Could you check a few things on this model? Use its own coordinates, in mm. Give positions to 0.01 mm unless a question says otherwise; leave off trailing zeros. Write each loop counter-clockwise with the first axis right and the second up, starting at its lowest first coordinate (ties: lowest second). Pieces come first, ordered by that corner, then holes. Notation, with made-up numbers: (70.5, 68) -> (114.5, 68) arc R19 cw to (114.5, 79) -> close; hole circle Ø8 at (13, -24). An arc over 180 degrees is marked (long way). One line per question, with ' | ' between items.
from build123d import *

# Parameters (mm, degrees)
SKETCH_1_W          = 60
SKETCH_1_H          = 18
EXTRUDE_1_DEPTH     = 11
SKETCH_2_R          = 1.55
CUT_EXTRUDE_2_DEPTH = 37.674241642


with BuildPart() as part:
    # 草图1 → 凸台-拉伸1 (new body)
    with BuildSketch(Plane(origin=(0, 0, 0), x_dir=(1, 0, 0), z_dir=(0, 1, 0))):
        Rectangle(SKETCH_1_W, SKETCH_1_H)
    extrude(amount=EXTRUDE_1_DEPTH)

    # 草图2 → 切除-拉伸2 (cut, through all)
    with BuildSketch(Plane.XY.offset(9)):
        with Locations((-24, 5.5)):
            Circle(SKETCH_2_R)
        with Locations((-18, 5.5)):
            Circle(SKETCH_2_R)
        with Locations((-12, 5.5)):
            Circle(SKETCH_2_R)
        with Locations((-6, 5.5)):
            Circle(SKETCH_2_R)
        with Locations((0, 5.5)):
            Circle(SKETCH_2_R)
        with Locations((6, 5.5)):
            Circle(SKETCH_2_R)
        with Locations((12, 5.5)):
            Circle(SKETCH_2_R)
        with Locations((18, 5.5)):
            Circle(SKETCH_2_R)
        with Locations((24, 5.5)):
            Circle(SKETCH_2_R)
    extrude(amount=-CUT_EXTRUDE_2_DEPTH, mode=Mode.SUBTRACT)


solid = part.part
Q1. Imagine slicing it at B-B on x = 12. Please give me the cut outline in (y, z).
Answer below:
outline: (0, -9) -> (3.95, -9) -> (3.95, 9) -> (0, 9) -> close; (7.05, -9) -> (11, -9) -> (11, 9) -> (7.05, 9) -> close
Q2. Will these pins go through, and if not, where does the flat tip stop? pin 1 (3 mm diameter, centred on x = -18, y = 5.5, fed in from +Z); pin 2 (3.5 mm diameter, centred on x = 0, y = 5.5, fed in from -Z).
Answer below:
pin 1: passes through | pin 2: stops at z = -9
Q3. If I drill on line 1 along Y through (x, z) = (-18, 3); line 2 along Y through (x, z) = (25, -2.75), over which ranges is the centre line in solid material (lowest first)?
Answer below:
line 1: y = 0 to 3.95, 7.05 to 11 | line 2: y = 0 to 4.32, 6.68 to 11
Q4. If we mould it in two halves opening along X, with no side actions, what happens to faces 1 (the flat face through (0, 3, 9)), 2 (the flat face through (-30, 5, 0)), 3 (the cylindrical face through (-0.202, 7.037, 0.126)), 4 (the cylindrical face through (-13.55, 5.57, 0.13))? For each: +X half, -X half, draft (parallel to the pull), parting line (faces both ways), or undercut.
Answer below:
face 1: draft | face 2: -X half | face 3: undercut | face 4: undercut
Q5. Imagine slicing it at A-A on z = 1.75. Count the separate pieces of the cut face and the enclosed holes in it, and give its area (3 significant figures).
Answer below:
separate pieces: 1 | enclosed holes: 9 | area: 592 mm^2
